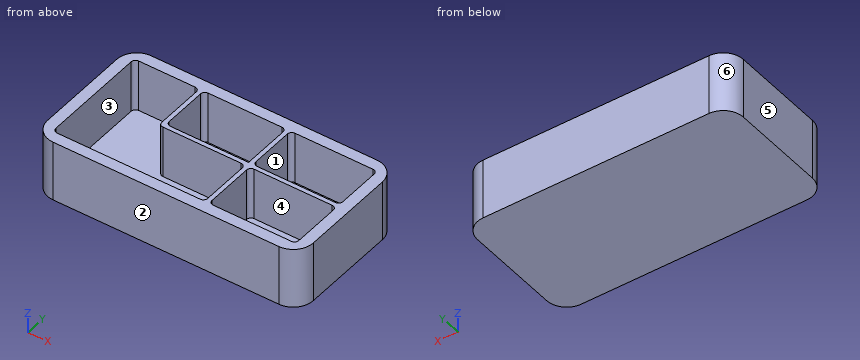
Autodesk Inventor part; units mm, degrees
ref_plane "YZ Plane" through (0, 0, 0) normal (1, 0, 0) x (0, 1, 0)
ref_plane "XZ Plane" through (0, 0, 0) normal (0, 1, 0) x (-1, 0, 0)
ref_plane "XY Plane" through (0, 0, 0) normal (0, 0, 1) x (1, 0, 0)
sketch "Esboço4" plane through (0, 0, 0) normal (0, 0, 1) x (1, 0, 0)
  line L0 (-130, -75) -> (130, -75)
  line L1 (150, -55) -> (150, 55)
  line L2 (130, 75) -> (-130, 75)
  line L3 (-150, 55) -> (-150, -55)
  line L4 (-150, -75) -> (150, 75) construction
  line L5 (150, -75) -> (-150, 75) construction
  arc A0 (-130, 75) -> (-150, 55) centre (-130, 55) ccw
  arc A1 (-150, -55) -> (-130, -75) centre (-130, -55) ccw
  arc A2 (130, -75) -> (150, -55) centre (130, -55) ccw
  arc A3 (150, 55) -> (130, 75) centre (130, 55) ccw
  line L6 (-153, -55) -> (-153, 55)
  arc A4 (-130, 78) -> (-153, 55) centre (-130, 55) ccw
  line L7 (-130, 78) -> (130, 78)
  arc A5 (153, 55) -> (130, 78) centre (130, 55) ccw
  line L8 (153, 55) -> (153, -55)
  arc A6 (130, -78) -> (153, -55) centre (130, -55) ccw
  line L9 (130, -78) -> (-130, -78)
  arc A7 (-153, -55) -> (-130, -78) centre (-130, -55) ccw
  line L10 (45, 65) -> (135, 65)
  line L11 (140, 60) -> (140, 10)
  line L12 (135, 5) -> (45, 5)
  line L13 (40, 10) -> (40, 60)
  line L14 (135, 70) -> (35, 70)
  line L15 (35, 60) -> (35, 5)
  line L16 (45, 0) -> (135, 0)
  line L17 (145, -5) -> (145, 60)
  line L18 (40, 0) -> (140, 0)
  line L19 (145, -5) -> (145, -60)
  line L20 (135, -70) -> (30, -70)
  line L21 (35, -60) -> (35, -5)
  line L22 (140, -5) -> (140, -60)
  line L23 (135, -65) -> (45, -65)
  line L24 (40, -60) -> (40, -5)
  line L25 (35, 70) -> (-70, 70)
  line L26 (-65, 60) -> (-65, 5)
  line L27 (-60, 0) -> (30, 0)
  line L28 (35, 5) -> (-55, 5)
  line L29 (-60, 10) -> (-60, 60)
  line L30 (-55, 65) -> (30, 65)
  line L31 (30, -70) -> (-135, -70)
  line L32 (-145, -60) -> (-145, 60)
  line L33 (-135, 70) -> (-70, 70)
  line L34 (-70, 65) -> (-135, 65)
  line L35 (-140, 60) -> (-140, -60)
  line L36 (-135, -65) -> (30, -65)
  arc A8 (135, -70) -> (145, -60) centre (135, -60) ccw
  arc A9 (145, 60) -> (135, 70) centre (135, 60) ccw
  arc A10 (-135, 70) -> (-145, 60) centre (-135, 60) ccw
  arc A11 (-145, -60) -> (-135, -70) centre (-135, -60) ccw
  arc A12 (-65, 5) -> (-60, 0) centre (-60, 5) ccw
  arc A13 (-60, 10) -> (-55, 5) centre (-55, 10) ccw
  arc A14 (40, 10) -> (45, 5) centre (45, 10) ccw
  arc A15 (35, -5) -> (30, 0) centre (30, -5) ccw
  arc A16 (45, 0) -> (40, -5) centre (45, -5) ccw
  arc A17 (35, 60) -> (30, 65) centre (30, 60) ccw
  arc A18 (45, 65) -> (40, 60) centre (45, 60) ccw
  arc A19 (-55, 65) -> (-60, 60) centre (-55, 60) ccw
  arc A20 (-65, 60) -> (-70, 65) centre (-70, 60) ccw
  arc A21 (140, 60) -> (135, 65) centre (135, 60) ccw
  arc A22 (135, 5) -> (140, 10) centre (135, 10) ccw
  arc A23 (140, -5) -> (135, 0) centre (135, -5) ccw
  arc A24 (135, -65) -> (140, -60) centre (135, -60) ccw
  arc A25 (40, -60) -> (45, -65) centre (45, -60) ccw
  arc A26 (30, -65) -> (35, -60) centre (30, -60) ccw
  arc A27 (-140, -60) -> (-135, -65) centre (-135, -60) ccw
  arc A28 (-135, 65) -> (-140, 60) centre (-135, 60) ccw
  point P0 (0, 0)
  point P1 (40, 65)
  point P2 (140, 5)
  point P3 (140, 65)
  point P4 (40, 5)
  point P5 (35, 0)
  point P6 (140, -65)
  point P7 (40, -65)
  point P8 (-65, 0)
  point P9 (-60, 5)
  point P10 (-60, 65)
  point P11 (-140, 65)
  point P12 (-140, -65)
  point P13 (35, 65)
  point P14 (35, -65)
  point P15 (-65, 65)
  point P16 (35, -11.1171)
  dimension "d13" = 150
  dimension "d14" = 300
  dimension "d17" = 20
  dimension "d18" = 20
  dimension "d19" = 3
  dimension "d20" = 60
  dimension "d21" = 100
  dimension "d25" = 5
  dimension "d26" = 5
  dimension "d27" = 5
  dimension "d28" = 5
  dimension "d31" = 5
  dimension "d32" = 5
  dimension "d33" = 5
  dimension "d38" = 100
  dimension "d39" = 5
  dimension "d41" = 5
  dimension "d42" = 5
  dimension "d43" = 5
  dimension "d44" = 5
  dimension "d47" = 5
  dimension "d49" = 100
  dimension "d50" = 5
  dimension "d57" = 10
  dimension "d62" = 60
  dimension "d63" = 5
  dimension "d64" = 5
extrude "Extrusão4" add sketch "Esboço4" along normal blind 60 contours A1 L3 A0 L2 A3 L1 A2 L0 | L6 A4 L7 A5 L8 A6 L9 A7 | L10 A21 L11 A22 L12 A14 L13 A18 | A9 L17 L19 A8 L20 L31 A11 L32 A10 L33 L25 L14 | L15 L28 A13 L29 A19 L30 A17 | L16 A23 L22 A24 L23 A25 L24 A16 | A26 L36 A27 L35 A28 L34 A20 L26 A12 L27 A15 L21
extrude "Extrusão5" cut sketch "Esboço4" along normal blind 80 contours L10 A21 L11 A22 L12 A14 L13 A18 | L15 L28 A13 L29 A19 L30 A17 | L16 A23 L22 A24 L23 A25 L24 A16 | A26 L36 A27 L35 A28 L34 A20 L26 A12 L27 A15 L21
extrude "Extrusão6" add sketch "Esboço4" against normal blind 10 contours A1 L3 A0 L2 A3 L1 A2 L0 | L6 A4 L7 A5 L8 A6 L9 A7 | L10 A21 L11 A22 L12 A14 L13 A18 | A9 L17 L19 A8 L20 L31 A11 L32 A10 L33 L25 L14 | L15 L28 A13 L29 A19 L30 A17 | L16 A23 L22 A24 L23 A25 L24 A16 | A26 L36 A27 L35 A28 L34 A20 L26 A12 L27 A15 L21
sketch "Esboço1" plane through (0, 0, 0) normal (0, 0, 1) x (1, 0, 0)
  line L0 (-25, -12.5) -> (25, -12.5)
  line L1 (25, -12.5) -> (25, 12.5)
  line L2 (25, 12.5) -> (-25, 12.5)
  line L3 (-25, 12.5) -> (-25, -12.5)
  line L4 (-25, -12.5) -> (25, 12.5) construction
  line L5 (25, -12.5) -> (-25, 12.5) construction
  point P0 (0, 0)
  dimension "d0" = 25
  dimension "d1" = 50
sketch "Esboço2" plane through (0, 0, 100) normal (0, 0, 1) x (1, 0, 0)
  line L0 (25, -12.5) -> (25, 12.5)
  line L1 (25, 12.5) -> (-25, 12.5)
  line L2 (-25, 12.5) -> (-25, -12.5)
  line L3 (-25, -12.5) -> (25, -12.5)
  line L4 (-27, 14.5) -> (27, 14.5)
  line L5 (27, 14.5) -> (27, -14.5)
  line L6 (27, -14.5) -> (-27, -14.5)
  line L7 (-27, -14.5) -> (-27, 14.5)
  point P0 (0, 0)
  dimension "d4" = 2
properties part number "prototipo"
CAD build for the part. Positions are in the model's coordinates, mm. Face numbers are marked on the shaded views. A direction names the side the tool comes from. Give positions to 0.01 mm unless a question says otherwise; leave off trailing zeros. Write each loop counter-clockwise with the first axis right and the second up, starting at its lowest first coordinate (ties: lowest second). Pieces come first, ordered by that corner, then holes. Notation, with made-up numbers: (78, 18) -> (88, 18) arc R27 cw to (88, 40) -> close; hole circle Ø3 at (47.5, 52). An arc over 180 degrees is marked (long way). Return JSON: item names as keys, results as strings.
Item 1: Band-saw the part on D-D (z = 22.5). Give the number of separate pieces and of enclosed holes in the cut face, then the cut area to 3 significant figures.
Answer below:
{"separate pieces": "1", "enclosed holes": "4", "area": "12,900 mm2"}
Item 2: Band-saw the part on B-B (y = 22). List the corners of the cut face in (x, z), then the cut area to 3 significant figures.
Answer below:
{"outline": "(-153, -10) -> (153, -10) -> (153, 60) -> (140, 60) -> (140, 0) -> (40, 0) -> (40, 60) -> (35, 60) -> (35, 0) -> (-60, 0) -> (-60, 60) -> (-65, 60) -> (-65, 0) -> (-140, 0) -> (-140, 60) -> (-153, 60) -> close", "area": "5,220 mm2"}
Item 3: Drop a flat-ended pin along its axis: pin 1 (18 mm diameter, centred on x = 66.5, y = 22.5, fed in from +Z). Give the stop position or say it passes through.
Answer below:
{"pin 1": "stops at z = 0"}
Item 4: Band-saw the part on C-C (x = 70). List the corners of the cut face in (y, z).
Answer below:
{"outline": "(-78, -10) -> (78, -10) -> (78, 60) -> (65, 60) -> (65, 0) -> (5, 0) -> (5, 60) -> (0, 60) -> (0, 0) -> (-65, 0) -> (-65, 60) -> (-78, 60) -> close"}
Item 5: Two-plate mould, pull along Y, no slides. Class the marked faces 3, 4, 5 and 6: +Y half, -Y half, draft (parallel to the pull), parting line (faces both ways), or undercut.
Answer below:
{"face 3": "undercut", "face 4": "undercut", "face 5": "draft", "face 6": "+Y half"}
Item 6: Drill centre lines: probe 1 along Y at (x, z) = (71, 48.5); probe 2 along X at (y, z) = (26.5, 37.5); probe 3 along X at (y, z) = (-54.5, 10.5). Where is each one in solid material? Low to high.
Answer below:
{"probe 1": "y = -78 to -65, 0 to 5, 65 to 78", "probe 2": "x = -153 to -140, -65 to -60, 35 to 40, 140 to 153", "probe 3": "x = -153 to -140, 35 to 40, 140 to 153"}
Item 7: Tool access for the marked faces 1 and 2: list every direction of +Z, -Z, +X, -X, +Y, -Y with a clear straight run to the whole face (end or side of a thin tool).
Answer below:
{"face 1": "+Z", "face 2": "+Z, -Z, +X, -X, -Y"}
Item 8: Band-saw the part on A-A (x = -86). List the corners of the cut face in (y, z).
Answer below:
{"outline": "(-78, -10) -> (78, -10) -> (78, 60) -> (65, 60) -> (65, 0) -> (-65, 0) -> (-65, 60) -> (-78, 60) -> close"}
